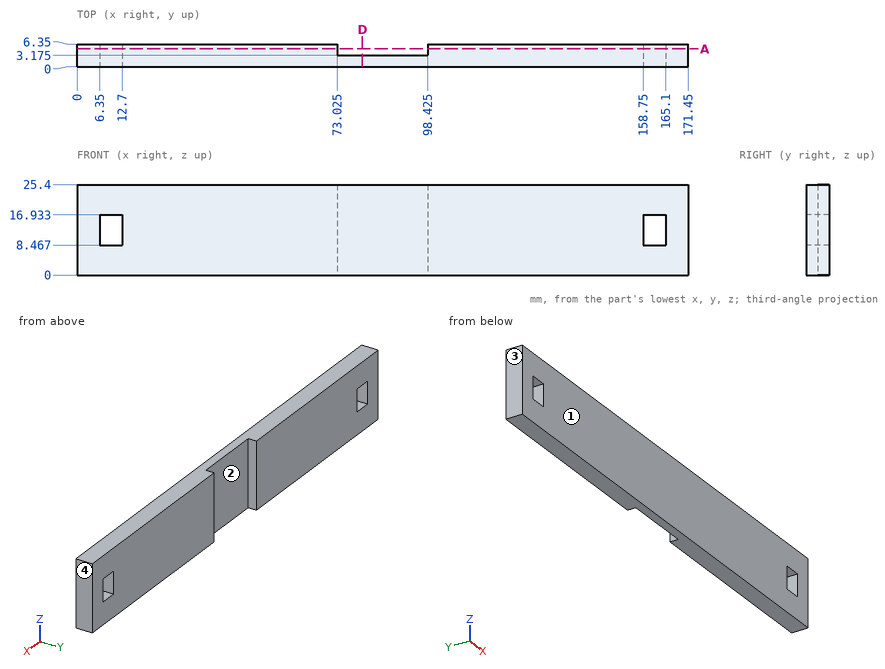
Design review of the part shown in the three views and the two pictorial views. Dimensions are in mm from the part's minimum x, y and z. Give positions to 0.01 mm unless a question says otherwise; leave off trailing zeros. Write each loop counter-clockwise with the first axis right and the second up, starting at its lowest first coordinate (ties: lowest second). Pieces come first, ordered by that corner, then holes. Notation, with made-up numbers: (-3.5, -37) - (39.5, -37) arc R19 ccw to (39.5, -10) - close; hole circle Ø4 at (86.25, 62). An arc over 180 degrees is marked (long way). Return JSON: item names as keys, results as strings. Group by question number.
(1) To check wall thickness, follow probe 1 along X at (y, z) = (2, 14.25); probe 2 along Z at (x, y) = (164, 0.5). State the ranges of each line that lie inside material, in increasing order.
(2) We need section A-A, the plane y = 5. Give the number of separate pieces and of enclosed holes in the cut face, then the cut area to 3 significant figures.
(3) Insertion check: pin 1 (2 mm diameter, centred on x = 19, y = 2, fed in from -Z); pin 2 (12.5 mm diameter, centred on x = 81, z = 9, fed in from +Y) (3 decimals). Each pin has a flat end and moves straight along its axis. Give the tip position at first contact, or say it passes through.
(4) We need section D-D, the plane x = 80. Give the boundary of the cut face in (y, z) (1 decimal).
(5) Mouldability with a two-part tool opening along X and no side actions: class the marked faces 1, 2, 3 and 4 as +X half, -X half, draft (parallel to the pull), parting line (faces both ways), or undercut.
Reported:
{
 "1": {"probe 1": "x = 0 to 6.35, 12.7 to 158.75, 165.1 to 171.45", "probe 2": "z = 0 to 8.47, 16.93 to 25.4"},
 "2": {"separate pieces": "2", "enclosed holes": "2", "area": "3,600 mm2"},
 "3": {"pin 1": "stops at z = 0", "pin 2": "stops at y = 3.175"},
 "4": {"outline": "(0, 0) - (3.2, 0) - (3.2, 25.4) - (0, 25.4) - close"},
 "5": {"face 1": "draft", "face 2": "undercut", "face 3": "-X half", "face 4": "+X half"}
}
